CAD build for the part. Positions are in the model's coordinates, mm. Round coordinates to 2 decimals unless told otherwise and drop trailing zeros. Loops run counter-clockwise (first coordinate to the right, second up) from the corner with the lowest first, then second, coordinate; pieces in that order, holes last. Notation, with made-up numbers: (54.5, -1.75) - (102.5, -1.75) arc R21 ccw to (102.5, 23.25) - close; hole circle Ø10 at (15, 46). An arc over 180 degrees is marked (long way). Use one line per item in the form item = value.
from build123d import *

# Parameters (mm, degrees)
SKETCH1_W               = 139
SKETCH1_H               = 6
BOSS_EXTRUDE1_DEPTH     = 1.38
CUT_EXTRUDE4_DEPTH      = 70.619448432
CUT_EXTRUDE4_DEPTH_BACK = 70.619448432
SKETCH8_R               = 1.7
CHAMFER2_SIZE           = 2


with BuildPart() as part:
    # Sketch1 → Boss-Extrude1 (new, symmetric)
    with BuildSketch(Plane(origin=(0, 0, 0), x_dir=(1, 0, 0), z_dir=(0, 1, 0))):
        Rectangle(SKETCH1_W, SKETCH1_H)
    extrude(amount=BOSS_EXTRUDE1_DEPTH, both=True)

    # Sketch8 → Cut-Extrude4 (cut, two sides: drawn at the far end of the back side and taken through both)
    with BuildSketch(Plane(origin=(0, 1.38, 0), x_dir=(1, 0, 0), z_dir=(0, 1, 0)).offset(-CUT_EXTRUDE4_DEPTH_BACK)):
        with Locations(Location((65, 0, 0), (0, 0, 270))):
            Circle(SKETCH8_R)
        with Locations(Location((-65, 0, 0), (0, 0, 270))):
            Circle(SKETCH8_R)
    extrude(amount=CUT_EXTRUDE4_DEPTH + CUT_EXTRUDE4_DEPTH_BACK, mode=Mode.SUBTRACT)

    # Chamfer2
    chamfer2_edges = [part.edges().sort_by_distance(p)[0] for p in [
        (69.5, 0, 3),
        (-69.5, 0, 3),
        (-69.5, 0, -3),
        (69.5, 0, -3),
    ]]
    chamfer(chamfer2_edges, length=CHAMFER2_SIZE)


solid = part.part
1) Slice it at B-B (z = 0). Write the cut outline in (x, y), plus the area to 3 significant figures.
Report:
outline = (-69.5, -1.38) - (-66.7, -1.38) - (-66.7, 1.38) - (-69.5, 1.38) - close; (-63.3, -1.38) - (63.3, -1.38) - (63.3, 1.38) - (-63.3, 1.38) - close; (66.7, -1.38) - (69.5, -1.38) - (69.5, 1.38) - (66.7, 1.38) - close
area = 365 mm^2
2) Drill centre lines: probe 1 along X at (y, z) = (-0.6, 0); probe 2 along Z at (x, y) = (-65, 0.7); probe 3 along X at (y, z) = (-0.85, 0.7). Where is each one in solid material? Low to high.
Report:
probe_1 = -69.5 to -66.7, -63.3 to 63.3, 66.7 to 69.5
probe_2 = -3 to -1.7, 1.7 to 3
probe_3 = -69.5 to -66.55, -63.45 to 63.45, 66.55 to 69.5
3) Slice it at A-A (x = 65). Write the cut outline in (y, z), plus the area to 3 significant figures.
Report:
outline = (-1.38, -3) - (1.38, -3) - (1.38, -1.7) - (-1.38, -1.7) - close; (-1.38, 1.7) - (1.38, 1.7) - (1.38, 3) - (-1.38, 3) - close
area = 7.18 mm^2
4) Slice it at C-C (y = -0.1). Write the cut outline in (x, z).
Report:
outline = (-69.5, -1) - (-67.5, -3) - (67.5, -3) - (69.5, -1) - (69.5, 1) - (67.5, 3) - (-67.5, 3) - (-69.5, 1) - close; hole circle Ø3.4 at (-65, 0); hole circle Ø3.4 at (65, 0)
5) Two-plate mould, pull along X, no slides. Class faces 1 (the cylindrical face through (66.15, -0.02, -1.25)), 2 (the flat face through (-1, 1.38, 0)): +X half, -X half, draft (parallel to the pull), parting line (faces both ways), or undercut.
Report:
face_1 = undercut
face_2 = draft
6) Flat gauge pin, fed straight in: pin 1 (2 mm diameter, centred on x = -65, z = 0, fed in from -Y). Where does the tip first touch, or does it go through?
Report:
pin_1 = through
